Source: CAD feature listing. Evaluate the final solid. Frame: model axes, mm. A direction names the side the tool comes from. Give positions to 0.01 mm unless a question says otherwise; leave off trailing zeros. Order: outer loops, then holes, each group sorted by start corner. A loop starts at its lowest first (then second) coordinate and runs counter-clockwise, first axis right, second up. Notation, with made-up numbers: M 3.5,-3.75 L 11.5,-3.75 A12 ccw 11.5,13.25 Z; hole C 84.5,3 d5. An arc over 180 degrees is marked long. Answer as a JSON object with one key per item and string values. Group by question number.
1. Section query D-D (y = -5). Output: boundary loops of the cut face in (x, z), plus the area to 3 significant figures.
2. Pin query (flat end, axial travel): P1, Ø1.5, axis at x = 31.5, z = -1.5, coming from the +Y side. Return the tip coordinate at first contact, or that it passes through.
3. Set-up query: faces 1 (the flat face through (37.63, -13.44, -1.03)), 2 (the flat face through (-22, -1, -1)), 3 (the flat face through (1, -10, -1)). Return all of +Z, -Z, +X, -X, +Y, -Y with unobstructed straight access to the full face (end or side cutting, diameter ignored); none if empty.
4. Material intervals for L1, parallel to Y at x = -23.5, z = -0.9; L2, parallel to X at y = -5.25, z = 0.8; L3, parallel to X at y = -4.75, z = 0.2, sorted ascending. Write a range as [from, to].
5. Section query C-C (y = 5). Output: boundary loops of the cut face in (x, z), plus the area to 3 significant figures.
6. Pull-direction query (X, two-part tool) for faces 4 (the flat face through (-1, -11, 1)), 5 (the flat face through (24, -1, -1)), 6 (the flat face through (-44.93, -16.154, -1.028)); classes: +X half, -X half, draft (parallel to the pull), parting line (faces both ways), or undercut.
7. Section query A-A (x = 40.5). Output: boundary loops of the cut face in (y, z).
8. Section query B-B (z = -1.35). Output: boundary loops of the cut face in (x, y).
from build123d import *

# Parameters (mm, degrees)
SKETCH005_R   = 2
SKETCH005_R_2 = 2.65
PAD_DEPTH     = 4


with BuildPart() as part:
    # Sketch005 → Pad (new body)
    with BuildSketch(Plane.XY.offset(-3)):
        Polygon((-25, 10), (-19, 10), (-19, 1), (-25, 1), (-25, -1), (-19, -1), (-19, -10), (21, -10), (21, -1), (27, -1), (27, 1), (21, 1), (21, 10), (28, 10), (47, 0.7), (47, -8.030345), (28, -19), (-40, -19), (-50, -13.226497), (-50, -6), align=None)
        with Locations((-23.5, 5)):
            Circle(SKETCH005_R, mode=Mode.SUBTRACT)
        with Locations((-23.5, -5)):
            Circle(SKETCH005_R, mode=Mode.SUBTRACT)
        with Locations((25.5, 5)):
            Circle(SKETCH005_R, mode=Mode.SUBTRACT)
        with Locations((25.5, -5)):
            Circle(SKETCH005_R, mode=Mode.SUBTRACT)
        with Locations((40.5, -5)):
            Circle(SKETCH005_R_2, mode=Mode.SUBTRACT)
        with Locations((-44.5, -10)):
            Circle(SKETCH005_R_2, mode=Mode.SUBTRACT)
    extrude(amount=PAD_DEPTH)


solid = part.part
Answer sheet:
{
 "1": {"outline": "M -48.44,-3 L -25.5,-3 L -25.5,1 L -48.44,1 Z; M -21.5,-3 L -19,-3 L -19,1 L -21.5,1 Z; M 21,-3 L 23.5,-3 L 23.5,1 L 21,1 Z; M 27.5,-3 L 37.85,-3 L 37.85,1 L 27.5,1 Z; M 43.15,-3 L 47,-3 L 47,1 L 43.15,1 Z", "area": "169 mm^2"},
 "2": {"P1": "y = 8.65"},
 "3": {"face 1": "+Z, -Z, +X, -Y", "face 2": "+Z, -Z", "face 3": "+Z, -Z, +Y"},
 "4": {"L1": "[-19, -7], [-3, -1], [1, 3], [7, 10]", "L2": "[-48.83, -25.48], [-21.52, -19], [21, 23.52], [27.48, 37.86], [43.14, 47]", "L3": "[-48.05, -25.48], [-21.52, -19], [21, 23.52], [27.48, 37.86], [43.14, 47]"},
 "5": {"outline": "M -32.81,-3 L -25.5,-3 L -25.5,1 L -32.81,1 Z; M -21.5,-3 L -19,-3 L -19,1 L -21.5,1 Z; M 21,-3 L 23.5,-3 L 23.5,1 L 21,1 Z; M 27.5,-3 L 38.22,-3 L 38.22,1 L 27.5,1 Z", "area": "92.1 mm^2"},
 "6": {"face 4": "draft", "face 5": "undercut", "face 6": "-X half"},
 "7": {"outline": "M -11.78,-3 L -7.65,-3 L -7.65,1 L -11.78,1 Z; M -2.35,-3 L 3.88,-3 L 3.88,1 L -2.35,1 Z"},
 "8": {"outline": "M -50,-13.23 L -40,-19 L 28,-19 L 47,-8.03 L 47,0.7 L 28,10 L 21,10 L 21,1 L 27,1 L 27,-1 L 21,-1 L 21,-10 L -19,-10 L -19,-1 L -25,-1 L -25,1 L -19,1 L -19,10 L -25,10 L -50,-6 Z; hole C -44.5,-10 d5.3; hole C -23.5,-5 d4; hole C -23.5,5 d4; hole C 25.5,-5 d4; hole C 25.5,5 d4; hole C 40.5,-5 d5.3"}
}
